```python
from build123d import *

# Parameters (mm, degrees)
SKETCH_1_W          = 48
SKETCH_1_H          = 24
EXTRUDE_1_DEPTH     = 1.5
FILLET_1_R          = 2
SKETCH_2_R          = 11
EXTRUDE_2_DEPTH     = 7
SKETCH_3_W          = 11
SKETCH_3_H          = 13
EXTRUDE_3_DEPTH     = 5
SKETCH_4_R          = 2
CUT_EXTRUDE_1_DEPTH = 5
SKETCH_5_R          = 1
CUT_EXTRUDE_2_DEPTH = 7


with BuildPart() as part:
    # 草图1 → 凸台-拉伸1 (new body)
    with BuildSketch(Plane.XY):
        Rectangle(SKETCH_1_W, SKETCH_1_H)
    extrude(amount=EXTRUDE_1_DEPTH)

    # 圆角1
    fillet_1_edges = [part.edges().sort_by_distance(p)[0] for p in [
        (24, -12, 0.75),
        (-24, -12, 0.75),
        (-24, 12, 0.75),
        (24, 12, 0.75),
    ]]
    fillet(fillet_1_edges, radius=FILLET_1_R)

    # 草图2 → 凸台-拉伸2 (add)
    with BuildSketch(Plane.XY.offset(1.5)):
        with Locations((13, 0)):
            Circle(SKETCH_2_R)
    extrude(amount=EXTRUDE_2_DEPTH)

    # 草图3 → 凸台-拉伸3 (add)
    with BuildSketch(Plane(origin=(0, 0, 0), x_dir=(-1, 0, 0), z_dir=(0, 0, -1))):
        with Locations((23.5, 0)):
            Rectangle(SKETCH_3_W, SKETCH_3_H)
    extrude(amount=EXTRUDE_3_DEPTH)

    # 草图4 → 切除-拉伸1 (cut)
    with BuildSketch(Plane.XY.offset(1.5)):
        with Locations((-11, 8)):
            Circle(SKETCH_4_R)
        with Locations(Location((-11, -8, 0), (0, 0, 180))):
            Circle(SKETCH_4_R)
    extrude(amount=-CUT_EXTRUDE_1_DEPTH, mode=Mode.SUBTRACT)

    # 草图5 → 切除-拉伸2 (cut)
    with BuildSketch(Plane.XY.offset(8.5)):
        with Locations((13, 0)):
            Circle(SKETCH_5_R)
        with Locations((13, 3)):
            Circle(SKETCH_5_R)
        with Locations((7, 0)):
            Circle(SKETCH_5_R)
        with Locations((15.598076211, 1.5)):
            Circle(SKETCH_5_R)
        with Locations((15.598076211, -1.5)):
            Circle(SKETCH_5_R)
        with Locations((13, -3)):
            Circle(SKETCH_5_R)
        with Locations((10.401923789, -1.5)):
            Circle(SKETCH_5_R)
        with Locations((10.401923789, 1.5)):
            Circle(SKETCH_5_R)
        with Locations((8.757359313, 4.242640687)):
            Circle(SKETCH_5_R)
        with Locations((13, 6)):
            Circle(SKETCH_5_R)
        with Locations((17.242640687, 4.242640687)):
            Circle(SKETCH_5_R)
        with Locations((19, 0)):
            Circle(SKETCH_5_R)
        with Locations((17.242640687, -4.242640687)):
            Circle(SKETCH_5_R)
        with Locations((13, -6)):
            Circle(SKETCH_5_R)
        with Locations((8.757359313, -4.242640687)):
            Circle(SKETCH_5_R)
    extrude(amount=-CUT_EXTRUDE_2_DEPTH, mode=Mode.SUBTRACT)


solid = part.part
```
Geometry: final body of the model. Coordinates: model frame, mm. A direction names the side the tool comes from. Round coordinates to 2 decimals unless told otherwise and drop trailing zeros. Order: outer loops, then holes, each group sorted by start corner. A loop starts at its lowest first (then second) coordinate and runs counter-clockwise, first axis right, second up. Notation, with made-up numbers: (-30.5, 43.5) -> (-5.5, 43.5) arc R10 cw to (-5.5, 49.5) -> close; hole circle Ø9 at (73, 83.25). An arc over 180 degrees is marked (long way). Use one line per item in the form item = value. Start each with the question number.
1. Reachability of faces 1 (the face through (7, 0, 1.5)), 2 (the face through (-23.43, -11.4, 0.76)), 3 (the face through (-24, 0, 1)) from +Z, -Z, +X, -X, +Y, -Y: full face, straight path, thin tool, end or side. Return the list, or none.
2. Cut plane C-C (z = 7.5). Count the separate pieces of the cut face and the enclosed holes in it, then the cut area to 3 significant figures.
3. Cut plane A-A (x = -11). Return the cut outline in (y, z).
4. Cut plane D-D (x = 13). Return the cut outline in (y, z), then the cut area to 3 significant figures.
5. Line query: probe 1 along Y at (x, z) = (-11, 0.85); probe 2 along X at (y, z) = (2.25, 4.5); probe 3 along X at (y, z) = (4.5, 7.25). Output: solid intervals per line, ascending.
6. Pin query (flat end, axial travel): pin 1 Ø2.5 at (y, z) = (1, -3.5) entering from +X; pin 2 Ø0.8 at (y, z) = (-4.5, 1) entering from -X; pin 3 Ø2 at (x, z) = (7, -2.5) entering from -Y; pin 4 Ø1.6 at (x, y) = (10.4, 1.5) entering from -Z. Return the tip coordinate at first contact, or that it passes through.
7. Cut plane B-B (y = 8.75). Return the cut outline in (x, z), then the cut area to 3 significant figures.
Solution:
q1.face_1 = +Z
q1.face_2 = +Z, -Z, -X, -Y
q1.face_3 = +Z, -X, +Y, -Y
q2.separate_pieces = 1
q2.enclosed_holes = 15
q2.area = 333 mm^2
q3.outline = (-12, 0) -> (-10, 0) -> (-10, 1.5) -> (-12, 1.5) -> close; (-6, 0) -> (6, 0) -> (6, 1.5) -> (-6, 1.5) -> close; (10, 0) -> (12, 0) -> (12, 1.5) -> (10, 1.5) -> close
q4.outline = (-12, 0) -> (12, 0) -> (12, 1.5) -> (11, 1.5) -> (11, 8.5) -> (7, 8.5) -> (7, 1.5) -> (5, 1.5) -> (5, 8.5) -> (4, 8.5) -> (4, 1.5) -> (2, 1.5) -> (2, 8.5) -> (1, 8.5) -> (1, 1.5) -> (-1, 1.5) -> (-1, 8.5) -> (-2, 8.5) -> (-2, 1.5) -> (-4, 1.5) -> (-4, 8.5) -> (-5, 8.5) -> (-5, 1.5) -> (-7, 1.5) -> (-7, 8.5) -> (-11, 8.5) -> (-11, 1.5) -> (-12, 1.5) -> close
q4.area = 120 mm^2
q5.probe_1 = -12 to -10, -6 to 6, 10 to 12
q5.probe_2 = 2.23 to 9.74, 11.06 to 12.34, 13.66 to 14.94, 16.26 to 23.77
q5.probe_3 = 2.96 to 7.79, 9.72 to 16.28, 18.21 to 23.04
q6.pin_1 = -18
q6.pin_2 = -24
q6.pin_3 = through
q6.pin_4 = 0
q7.outline = (-24, 0) -> (-12.85, 0) -> (-12.85, 1.5) -> (-24, 1.5) -> close; (-9.15, 0) -> (24, 0) -> (24, 1.5) -> (19.67, 1.5) -> (19.67, 8.5) -> (6.33, 8.5) -> (6.33, 1.5) -> (-9.15, 1.5) -> close
q7.area = 160 mm^2
